Could you check a few things on this model? Use its own coordinates, in mm. A direction names the side the tool comes from. Coordinates: 2 decimals unless noted, no trailing zeros. Write each loop counter-clockwise with the first axis right and the second up, starting at its lowest first coordinate (ties: lowest second). Pieces come first, ordered by that corner, then holes. Notation, with made-up numbers: (64.5, -3.5) - (80.5, -3.5) arc R22 cw to (80.5, 35.5) - close; hole circle Ø3 at (28.5, -38.75). An arc over 180 degrees is marked (long way). Write item = value, one per line. Start each with the question number.
```python
from build123d import *

# Parameters (mm, degrees)
SKETCH1_W           = 20
SKETCH1_H           = 20
SKETCH1_W_2         = 18
SKETCH1_H_2         = 18
BOSS_EXTRUDE1_DEPTH = 66
SKETCH2_R           = 2.6
CUT_EXTRUDE1_DEPTH  = 66
SKETCH3_R           = 2.6
CUT_EXTRUDE2_DEPTH  = 66


with BuildPart() as part:
    # Sketch1 → Boss-Extrude1 (new body)
    with BuildSketch(Plane(origin=(0, 0, 0), x_dir=(1, 0, 0), z_dir=(0, 1, 0))):
        with Locations((10, 10)):
            Rectangle(SKETCH1_W, SKETCH1_H)
        with Locations((10, 10)):
            Rectangle(SKETCH1_W_2, SKETCH1_H_2, mode=Mode.SUBTRACT)
    extrude(amount=BOSS_EXTRUDE1_DEPTH)

    # Sketch2 → Cut-Extrude1 (cut)
    with BuildSketch(Plane(origin=(20, 0, 0), x_dir=(0, 0, -1), z_dir=(1, 0, 0))):
        with Locations((10, 55.2)):
            Circle(SKETCH2_R)
    extrude(amount=-CUT_EXTRUDE1_DEPTH, mode=Mode.SUBTRACT)

    # Sketch3 → Cut-Extrude2 (cut)
    with BuildSketch(Plane(origin=(0, 0, -20), x_dir=(-1, 0, 0), z_dir=(0, 0, -1))):
        with Locations((-10, 10.8)):
            Circle(SKETCH3_R)
    extrude(amount=-CUT_EXTRUDE2_DEPTH, mode=Mode.SUBTRACT)


solid = part.part
```
1) Suppose I cut it at B-B on x = 10. Please give me the cut outline in (y, z), plus the area to 3 significant figures.
2) Suppose I cut it at D-D on y = 24. Please give me the cut outline in (x, z), plus the area to 3 significant figures.
3) If I drill on probe 1 along X at (y, z) = (25, -11.5); probe 2 along Y at (x, z) = (0.6, -10); probe 3 along Y at (x, z) = (10, -0.65), over which ranges is the centre line in solid material (lowest first)? Write a range as [from, to].
4) Suppose I cut it at A-A on x = 6.25. Please give me the cut outline in (y, z), plus the area to 3 significant figures.
5) Suppose I cut it at C-C on z = -17. Please give me the cut outline in (x, y), plus the area to 3 significant figures.
6) Thinking about a two-plate mould opening in Z: for faces 3 (the flat face through (10, 33, 0)), 4 (the cylindrical face through (0.51, 52.66, -9.44)), 5 (the flat face through (0, 33, -10)), which applies, +Z half, -Z half, draft (parallel to the pull), parting line (faces both ways), or undercut?
7) Which directions (+Z, -Z, +X, -X, +Y, -Y) give clear straight access to the entire face, cutting with the end or side of a thin tool? Please do faces 1 (the flat face through (10, 33, -20)), 2 (the flat face through (10, 33, -19)).
Reply:
q1.outline = (0, -20) - (8.2, -20) - (8.2, -19) - (0, -19) - close; (0, -1) - (8.2, -1) - (8.2, 0) - (0, 0) - close; (13.4, -20) - (66, -20) - (66, -19) - (13.4, -19) - close; (13.4, -1) - (66, -1) - (66, 0) - (13.4, 0) - close
q1.area = 122 mm^2
q2.outline = (0, -20) - (20, -20) - (20, 0) - (0, 0) - close; hole (1, -19) - (19, -19) - (19, -1) - (1, -1) - close
q2.area = 76.0 mm^2
q3.probe_1 = [0, 1], [19, 20]
q3.probe_2 = [0, 52.6], [57.8, 66]
q3.probe_3 = [0, 8.2], [13.4, 66]
q4.outline = (0, -20) - (66, -20) - (66, -19) - (0, -19) - close; (0, -1) - (66, -1) - (66, 0) - (0, 0) - close
q4.area = 132 mm^2
q5.outline = (0, 0) - (1, 0) - (1, 66) - (0, 66) - close; (19, 0) - (20, 0) - (20, 66) - (19, 66) - close
q5.area = 132 mm^2
q6.face_3 = +Z half
q6.face_4 = undercut
q6.face_5 = draft
q7.face_1 = -Z, +X, -X, +Y, -Y
q7.face_2 = +Y, -Y
